Input: part model. Units: mm. Frame: model coordinates. A direction names the side the tool comes from. Round coordinates to 2 decimals unless told otherwise and drop trailing zeros. Loops run counter-clockwise (first coordinate to the right, second up) from the corner with the lowest first, then second, coordinate; pieces in that order, holes last.
1) Section A-A, the plane z = 7.5. Return loops of the section in (x, y), and give its area (3 significant figures).
2) Draft query along X for faces 4 (the face through (-68, 5.813, 82)), 5 (the face through (-51, 7.813, 44)), 6 (the face through (-89.247, 3, 2)), 7 (the face through (-69, 9, 85)). Return one class per face: pulls with the +X half, pulls with the -X half, needs draft (parallel to the pull), parting line crosses it, or undercut.
3) Ray query, line 1 along X through (y, z) = (5.5, 33); line 2 along Z through (x, y) = (-79.5, 3.75); line 3 along Z through (x, y) = (-68, 5.25). Return the intervals inside material, ascending.
4) First-contact query: pin 1 (4 mm diameter, centred on x = -49.5, z = 63, fed in from +Y); pin 2 (0.6 mm diameter, centred on x = -49, y = 1, fed in from +Z); pin 3 (1 mm diameter, centred on y = 1, z = 8.5, fed in from -X). Flat tips, straight axial feed; report the tip coordinate or a pass-through.
5) Section D-D, the plane z = 30. Return loops of the section in (x, y).
6) Section B-B, the plane y = 10.5. Return loops of the section in (x, z), and give its area (3 significant figures).
7) Access query for faces 1 (the face through (-69, 3, 0)), 2 (the face through (-65.997, 9, 82)), 3 (the face through (-87, 1.713, 10)). Directions: +Z, -Z, +X, -X, +Y, -Y. A direction counts if a zero-diameter tool reaches every point of the face in a straight line with its end or side. Return the directions, or none.
8) Section C-C, the plane x = -76. Return loops of the section in (y, z), and give its area (3 significant figures).
from build123d import *

# Parameters (mm, degrees)
F0_W      = 4.2
F0_H      = 1.2
F1_DEPTH  = 15
F0_W_2    = 32.7
F2_DEPTH  = 5
F4_DEPTH  = 5
F6_DEPTH  = 5
F7_W      = 9.5
F7_H      = 3
F8_DEPTH  = 90
F9_W      = 9.5
F9_H      = 3
F10_DEPTH = 15
F11_DEPTH = 10.1
F12_DEPTH = 5
F13_W     = 5
F13_H     = 5.1
F14_DEPTH = 4.5
F15_W     = 3
F15_H     = 3
F16_DEPTH = 90


with BuildPart() as f1:
    # F0 (on Top) → F1 (new body)
    with BuildSketch(Plane.XY):
        with Locations((-86.9470929563, 1.1125010281)):
            Rectangle(F0_W, F0_H)
    extrude(amount=F1_DEPTH)



with BuildPart() as f1b:
    # F0 (on Top) → F1, piece 2 (new body)
    with BuildSketch(Plane.XY):
        with Locations((-50.0470929563, 1.1125010281)):
            Rectangle(F0_W, F0_H)
    extrude(amount=F1_DEPTH)


with BuildPart() as f1_1:
    add(f1.part)

    add(f1b.part)  # F2 merges F1b
    # F0 (on Top) → F2 (join)
    with BuildSketch(Plane.XY):
        with Locations((-68.4970929563, 1.1125010281)):
            Rectangle(F0_W_2, F0_H)
    extrude(amount=F2_DEPTH)

    # F3 (on face) → F4 (join)
    with BuildSketch(Plane(origin=(0, 0, 0), x_dir=(1, 0, 0), z_dir=(0, 0, -1))):
        Polygon((-52.1470929563, -0.5125010281), (-84.8470929563, -0.5125010281), (-89.2470929563, -0.5125010281), (-89.2470929563, -4.8120530977), (-68.4970929563, -4.8593617954), (-47.7470929563, -4.8125010281), (-47.7470929563, -0.5125010281), align=None)
    extrude(amount=-F4_DEPTH)

    # F5: union 

    # F3 (on face) → F6 (join)
    with BuildSketch(Plane(origin=(0, 0, 0), x_dir=(1, 0, 0), z_dir=(0, 0, -1))):
        Polygon((-52.1470929563, -0.5125010281), (-84.8470929563, -0.5125010281), (-89.2470929563, -0.5125010281), (-89.2470929563, -4.8120530977), (-68.4970929563, -4.8593617954), (-47.7470929563, -4.8125010281), (-47.7470929563, -0.5125010281), align=None)
    extrude(amount=-F6_DEPTH)

    # F7 (on face) → F8 (join)
    with BuildSketch(Plane(origin=(0, 0, 0), x_dir=(1, 0, 0), z_dir=(0, 0, -1))):
        with Locations((-84.4970929563, -6.3120530977)):
            Rectangle(F7_W, F7_H)
        with Locations((-52.4970929563, -6.3125010281)):
            Rectangle(F7_W, F7_H)
    extrude(amount=-F8_DEPTH)

    # F9 (on face) → F10 (join)
    with BuildSketch(Plane.XY.offset(90)):
        Polygon((-89.2470929563, 4.8125010281), (-57.2470929563, 4.8125010281), (-57.2470929563, 7.8125010281), (-68.4970929563, 7.8125010281), (-89.2470929563, 7.8125010281), align=None)
        with Locations((-52.4970929563, 6.3125010281)):
            Rectangle(F9_W, F9_H)
        Polygon((-57.2470929563, 7.8125010281), (-47.7470929563, 7.8125010281), (-65.9970929563, 12.2100913895), (-65.9970929563, 10.3125010281), (-68.4970929563, 10.3125010281), (-68.4970929563, 7.8125010281), align=None)
        Polygon((-70.9970929563, 12.2100913895), (-89.2470929563, 7.8125010281), (-68.4970929563, 7.8125010281), (-68.4970929563, 10.3125010281), (-70.9970929563, 10.3125010281), align=None)
        Polygon((-68.4970929563, 10.3125010281), (-68.4970929563, 12.8125010281), (-70.9970929563, 12.2100913895), (-70.9970929563, 10.3125010281), align=None)
        Polygon((-65.9970929563, 10.3125010281), (-65.9970929563, 12.2100913895), (-68.4970929563, 12.8125010281), (-68.4970929563, 10.3125010281), align=None)
    extrude(amount=-F10_DEPTH)

    # F9 (on face) → F11 (cut)
    with BuildSketch(Plane.XY.offset(90)):
        Polygon((-68.4970929563, 10.3125010281), (-68.4970929563, 12.8125010281), (-70.9970929563, 12.2100913895), (-70.9970929563, 10.3125010281), align=None)
        Polygon((-65.9970929563, 10.3125010281), (-65.9970929563, 12.2100913895), (-68.4970929563, 12.8125010281), (-68.4970929563, 10.3125010281), align=None)
    extrude(amount=-F11_DEPTH, mode=Mode.SUBTRACT)

    # F9 (on face) → F12 (join)
    with BuildSketch(Plane.XY.offset(90)):
        Polygon((-65.9970929563, 10.3125010281), (-65.9970929563, 12.2100913895), (-68.4970929563, 12.8125010281), (-68.4970929563, 10.3125010281), align=None)
        Polygon((-68.4970929563, 10.3125010281), (-68.4970929563, 12.8125010281), (-70.9970929563, 12.2100913895), (-70.9970929563, 10.3125010281), align=None)
    extrude(amount=-F12_DEPTH)

    # F13 (on face) → F14 (cut)
    with BuildSketch(Plane(origin=(0, 10.3125010281, 0), x_dir=(-1, 0, 0), z_dir=(0, 1, 0))):
        with Locations((68.4970929563, 82.45)):
            Rectangle(F13_W, F13_H)
    extrude(amount=-F14_DEPTH, mode=Mode.SUBTRACT)

    # F15 (on face) → F16 (join)
    with BuildSketch(Plane(origin=(0, 0, 0), x_dir=(1, 0, 0), z_dir=(0, 0, -1))):
        with Locations((-46.2470929563, -6.3125010281)):
            Rectangle(F15_W, F15_H)
        with Locations((-90.7470929563, -6.3120530977)):
            Rectangle(F15_W, F15_H)
    extrude(amount=-F16_DEPTH)


solid = f1_1.part
Final values:
1. outline: (-92.25, 4.81) - (-79.75, 4.81) - (-79.75, 7.81) - (-92.25, 7.81) - close; (-89.05, 0.51) - (-84.85, 0.51) - (-84.85, 1.71) - (-89.05, 1.71) - close; (-57.25, 4.81) - (-44.75, 4.81) - (-44.75, 7.81) - (-57.25, 7.81) - close; (-52.15, 0.51) - (-47.95, 0.51) - (-47.95, 1.71) - (-52.15, 1.71) - close
1. area: 85.1 mm2
2. face 4: undercut
2. face 5: needs draft
2. face 6: pulls with the -X half
2. face 7: undercut
3. line 1: x = -92.25 to -79.75, -57.25 to -44.75
3. line 2: z = 0 to 5
3. line 3: z = 75 to 90
4. pin 1: stops at y = 7.81
4. pin 2: stops at z = 15
4. pin 3: stops at x = -89.05
5. outline: (-92.25, 4.81) - (-79.75, 4.81) - (-79.75, 7.81) - (-92.25, 7.81) - close; (-57.25, 4.81) - (-44.75, 4.81) - (-44.75, 7.81) - (-57.25, 7.81) - close
6. outline: (-78.09, 75) - (-58.9, 75) - (-58.9, 90) - (-78.09, 90) - close; hole (-71, 79.9) - (-66, 79.9) - (-66, 85) - (-71, 85) - close
6. area: 262 mm2
7. face 1: -Z, +X, -X, +Y, -Y
7. face 2: +Y
7. face 3: +Z, +X, -X
8. outline: (0.51, 0) - (4.84, 0) - (4.84, 5) - (0.51, 5) - close; (4.81, 75) - (11, 75) - (11, 90) - (4.81, 90) - close
8. area: 115 mm2
